Can you work these out from the model? Positions are in its coordinate system, mm. A direction names the side the tool comes from. Coordinates: 2 decimals unless noted, no trailing zeros. Write each loop counter-clockwise with the first axis right and the second up, starting at its lowest first coordinate (ties: lowest second). Pieces come first, ordered by that corner, then holes. Notation, with made-up numbers: M 72.5,73 L 118.5,73 A8 ccw 118.5,84 Z; hole C 22,87.25 d2. An arc over 180 degrees is marked long. Answer as a JSON object with one key per item and string values. Group by question number.
from build123d import *

# Parameters (mm, degrees)
F0_R     = 8.5
F1_DEPTH = 8


with BuildPart() as f1:
    # F0 (on Front) → F1 (new body)
    with BuildSketch(Plane.XZ):
        with BuildLine():
            Line((88.008557, 80.983967), (-79.72115, 80.983967))
            Line((-79.72115, 80.983967), (-79.72115, 30.726752))
            ThreePointArc((-79.72115, 30.726752), (-77.761317, 14.88575), (-72, 0))
            Line((-72, 0), (-52, 0))
            ThreePointArc((-52, 0), (-61.959604, 16.838163), (-48.181921, 30.726752))
            Line((-48.181921, 30.726752), (-26.181921, 30.726752))
            ThreePointArc((-26.181921, 30.726752), (-23.867446, 13.648604), (-12.537347, 0.662117))
            Line((-12.537347, 0.662117), (3.462653, 0.662117))
            ThreePointArc((3.462653, 0.662117), (-7.925971, 15.116443), (1.818079, 30.726752))
            Line((1.818079, 30.726752), (23.818079, 30.726752))
            ThreePointArc((23.818079, 30.726752), (26.923148, 12.938641), (39.676101, 0.155035))
            Line((39.676101, 0.155035), (55.676101, 0.155035))
            ThreePointArc((55.676101, 0.155035), (42.154292, 13.977932), (51.818079, 30.726752))
            Line((51.818079, 30.726752), (88.008557, 30.983967))
            Line((88.008557, 30.983967), (88.008557, 80.983967))
        make_face()
        with Locations((63.008557, 55.983967)):
            Circle(F0_R, mode=Mode.SUBTRACT)
    extrude(amount=F1_DEPTH)


solid = f1.part
Q1. If we section it at C-C on z = 28.5: List the corners of the cut face in (x, y) for me, and give its area (3 significant figures).
Q2. If we section it at D-D on z = 59.5: List the corners of the cut face in (x, y) for me.
Q3. If we section it at B-B on y = -3.5: List the corners of the cut face in (x, z) for me.
Q4. If we section it at A-A on x = 48: List the corners of the cut face in (y, z) for me.
Q5. On a 3-axis mill with a long thin cutter (end or side, diameter ignored), from which of +Z, -Z, +X, -X, +Y, -Y can I reach the whole of each face in a straight line? I mean faces 1 (the flat face through (48, -4, 0.155)), 2 (the flat face through (-5, -4, 0.662)), 3 (the cylindrical face through (-7.91, -3.94, 14.84)), 4 (the cylindrical face through (42.193, -3.944, 13.69)). Say none if no direction works.
Q6. Please list where these lines run through material, in increasing order: L1, parallel to X at y = -2, z = 14; L2, parallel to X at y = -4, z = 25.5; L3, parallel to Z at x = 4.5, y = -6.5.
Q7. We'd pull the mould along X, two halves only. Please class faces 5 (the flat face through (-79.721, -4, 56)), 6 (the cylindrical face through (26.806, -3.944, 13.167)), 7 (the flat face through (5, -4, 80.984)): pulls with the +X half, pulls with the -X half, needs draft (parallel to the pull), parting line crosses it, or undercut.
Q8. Will these pins go through, and if not, where does the flat tip stop? pin 1 (2.5 mm diameter, centred on x = -36, y = -2, fed in from -Z); pin 2 (1.5 mm diameter, centred on x = 37.5, y = -5, fed in from -Z).
Reply:
{
 "1": {"outline": "M -79.68,-8 L -54.45,-8 L -54.45,0 L -79.68,0 Z; M -26.45,-8 L -1.93,-8 L -1.93,0 L -26.45,0 Z; M 23.6,-8 L 48.06,-8 L 48.06,0 L 23.6,0 Z", "area": "594 mm^2"},
 "2": {"outline": "M -79.72,-8 L 55.27,-8 L 55.27,0 L -79.72,0 Z; M 70.75,-8 L 88.01,-8 L 88.01,0 L 70.75,0 Z"},
 "3": {"outline": "M -79.72,30.73 A65 ccw -72,0 L -52,0 A16 cw -48.18,30.73 L -26.18,30.73 A30 ccw -12.54,0.66 L 3.46,0.66 A16 cw 1.82,30.73 L 23.82,30.73 A30 ccw 39.68,0.16 L 55.68,0.16 A16 cw 51.82,30.73 L 88.01,30.98 L 88.01,80.98 L -79.72,80.98 Z; hole C 63.01,55.98 d17"},
 "4": {"outline": "M -8,0.16 L 0,0.16 L 0,3.51 L -8,3.51 Z; M -8,28.45 L 0,28.45 L 0,80.98 L -8,80.98 Z"},
 "5": {"face 1": "-Z, +X, +Y, -Y", "face 2": "-Z, +Y, -Y", "face 3": "+Y, -Y", "face 4": "+X, +Y, -Y"},
 "6": {"L1": "-77.53 to -62.06, -24.02 to -7.83, 26.4 to 42.15", "L2": "-79.51 to -58.04, -26.54 to -4.82, 23.58 to 45.17", "L3": "30.73 to 80.98"},
 "7": {"face 5": "pulls with the -X half", "face 6": "undercut", "face 7": "needs draft"},
 "8": {"pin 1": "z = 30.73", "pin 2": "z = 0.95"}
}
